```python
from build123d import *

# Parameters (mm, degrees)
ESBO_O1_W                = 20
ESBO_O1_H                = 25
RESSALTO_EXTRUS_O1_DEPTH = 3
ESBO_O2_W                = 15
ESBO_O2_H                = 5
RESSALTO_EXTRUS_O2_DEPTH = 7
FILETE3_R                = 3
ESBO_O4_W                = 8
ESBO_O4_H                = 3
CORTE_EXTRUS_O2_DEPTH    = 27.025134469
FILETE4_R                = 3


with BuildPart() as part:
    # Esboço1 → Ressalto-extrusão1 (new body)
    with BuildSketch(Plane(origin=(0, 0, 0), x_dir=(1, 0, 0), z_dir=(0, 1, 0))):
        Rectangle(ESBO_O1_W, ESBO_O1_H)
    extrude(amount=RESSALTO_EXTRUS_O1_DEPTH)

    # Esboço2 → Ressalto-extrusão2 (add)
    with BuildSketch(Plane(origin=(0, 0, 0), x_dir=(-1, 0, 0), z_dir=(0, -1, 0))):
        with Locations((0, 7.984943423)):
            Rectangle(ESBO_O2_W, ESBO_O2_H)
        with Locations((0, -7.984943423)):
            Rectangle(ESBO_O2_W, ESBO_O2_H)
    extrude(amount=RESSALTO_EXTRUS_O2_DEPTH)

    # Filete3
    filete3_edges = [part.edges().sort_by_distance(p)[0] for p in [
        (10, 1.5, 12.5),
        (-10, 1.5, 12.5),
        (-10, 1.5, -12.5),
        (10, 1.5, -12.5),
    ]]
    fillet(filete3_edges, radius=FILETE3_R)

    # Esboço4 → Corte-extrusão2 (cut, through all)
    with BuildSketch(Plane(origin=(0, 0, -10.484943423), x_dir=(-1, 0, 0), z_dir=(0, 0, -1))):
        with Locations((0, -2.5)):
            Rectangle(ESBO_O4_W, ESBO_O4_H)
    extrude(amount=-CORTE_EXTRUS_O2_DEPTH, mode=Mode.SUBTRACT)

    # Filete4
    filete4_edges = [part.edges().sort_by_distance(p)[0] for p in [
        (-7.5, -7, -7.984943423),
        (7.5, -7, -7.984943423),
        (7.5, -7, 7.984943423),
        (-7.5, -7, 7.984943423),
    ]]
    fillet(filete4_edges, radius=FILETE4_R)


solid = part.part
```
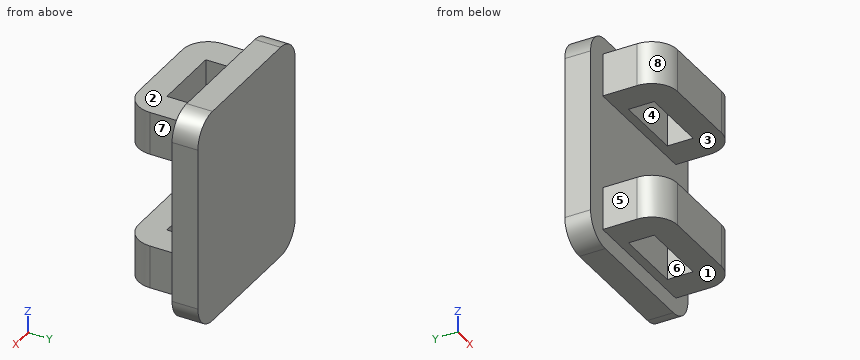
Geometry check sheet. Reference: the model listing, model coordinates, mm. Face numbers are marked on the shaded views. A direction names the side the tool comes from. Round coordinates to 2 decimals unless told otherwise and drop trailing zeros. Loops run counter-clockwise (first coordinate to the right, second up) from the corner with the lowest first, then second, coordinate; pieces in that order, holes last. Notation, with made-up numbers: M 48.5,84.5 L 92.5,84.5 A13 ccw 92.5,109.5 Z; hole C -30,-13.5 d1. An arc over 180 degrees is marked long. Return JSON: item names as keys, results as strings. Group by question number.
(1) Mould release check, pull along X, two halves, no side actions. Record for the marked faces 6, 7 and 8: pulls with the +X half, pulls with the -X half, needs draft (parallel to the pull), parting line crosses it, or undercut.
(2) Section check B-B, the plane y = -3.25. Enter the section's corners in (x, z), and give its area (3 significant figures).
(3) Section check A-A, the plane x = 1.75. Enter the section's corners in (y, z), and give its area (3 significant figures).
(4) Section check D-D, the plane z = -6.75. Enter the section's corners in (x, y), and give its area (3 significant figures).
(5) Set-up check for the marked faces 1, 2, 3, 4 and 5: record each of +Z, -Z, +X, -X, +Y, -Y from which the full face is reachable in a straight line by a thin tool's end or side.
(6) Scan lines: line 1 along Y through (x, z) = (-1.75, -10.25); line 2 along Z through (x, y) = (-3.75, -6); line 3 along X through (y, z) = (-2.5, -6.5). Record each from-to range of solid material in increasing order. Write a range as [from, to].
(7) Go/stop test with flat-tipped pins: pin 1 (4.5 mm diameter, centred on y = -3, z = 8.5, fed in from +X); pin 2 (3 mm diameter, centred on y = -3, z = 7, fed in from -X); pin 3 (3.5 mm diameter, centred on x = 1.5, y = -3, fed in from -Z). Record where each tip stops, or that it passes through.
(8) Section check C-C, the plane y = -0.5. Enter the section's corners in (x, z).
Data:
{
 "1": {"face 6": "undercut", "face 7": "pulls with the +X half", "face 8": "pulls with the -X half"},
 "2": {"outline": "M -7.5,-10.48 L -4,-10.48 L -4,-5.48 L -7.5,-5.48 Z; M -7.5,5.48 L -4,5.48 L -4,10.48 L -7.5,10.48 Z; M 4,-10.48 L 7.5,-10.48 L 7.5,-5.48 L 4,-5.48 Z; M 4,5.48 L 7.5,5.48 L 7.5,10.48 L 4,10.48 Z", "area": "70.0 mm²"},
 "3": {"outline": "M -7,-10.48 L -4,-10.48 L -4,-5.48 L -7,-5.48 Z; M -7,5.48 L -4,5.48 L -4,10.48 L -7,10.48 Z; M -1,-10.48 L 0,-10.48 L 0,-12.5 L 3,-12.5 L 3,12.5 L 0,12.5 L 0,10.48 L -1,10.48 L -1,5.48 L 0,5.48 L 0,-5.48 L -1,-5.48 Z", "area": "115 mm²"},
 "4": {"outline": "M -10,0 L -7.5,0 L -7.5,-4 A3 ccw -4.5,-7 L 4.5,-7 A3 ccw 7.5,-4 L 7.5,0 L 10,0 L 10,3 L -10,3 Z; hole M -4,-4 L 4,-4 L 4,-1 L -4,-1 Z", "area": "137 mm²"},
 "5": {"face 1": "-Z, +X, -X, -Y", "face 2": "+Z, +X, -X, -Y", "face 3": "+X, -X, -Y", "face 4": "+Z, -Z", "face 5": "+Z, -Z, -X, -Y"},
 "6": {"line 1": "[-7, -4], [-1, 3]", "line 2": "[-10.48, -5.48], [5.48, 10.48]", "line 3": "[-7.5, -4], [4, 7.5]"},
 "7": {"pin 1": "x = 7.5", "pin 2": "x = -7.5", "pin 3": "z = -10.48"},
 "8": {"outline": "M -7.5,-10.48 L 7.5,-10.48 L 7.5,-5.48 L -7.5,-5.48 Z; M -7.5,5.48 L 7.5,5.48 L 7.5,10.48 L -7.5,10.48 Z"}
}
